Here's the drawing with two shaded views (mm, measured from the low corner). I have some questions. A direction names the side the tool comes from. Give positions to 0.01 mm unless a question says otherwise; leave off trailing zeros. Loops run counter-clockwise (first coordinate to the right, second up) from the corner with the lowest first, then second, coordinate; pieces in that order, holes last. Notation, with made-up numbers: M 15.5,8 L 55.5,8 A18 cw 55.5,21 Z; hole C 45.5,61 d6. An arc over 180 degrees is marked long. Write item = value, one per line. Start each with the question number.
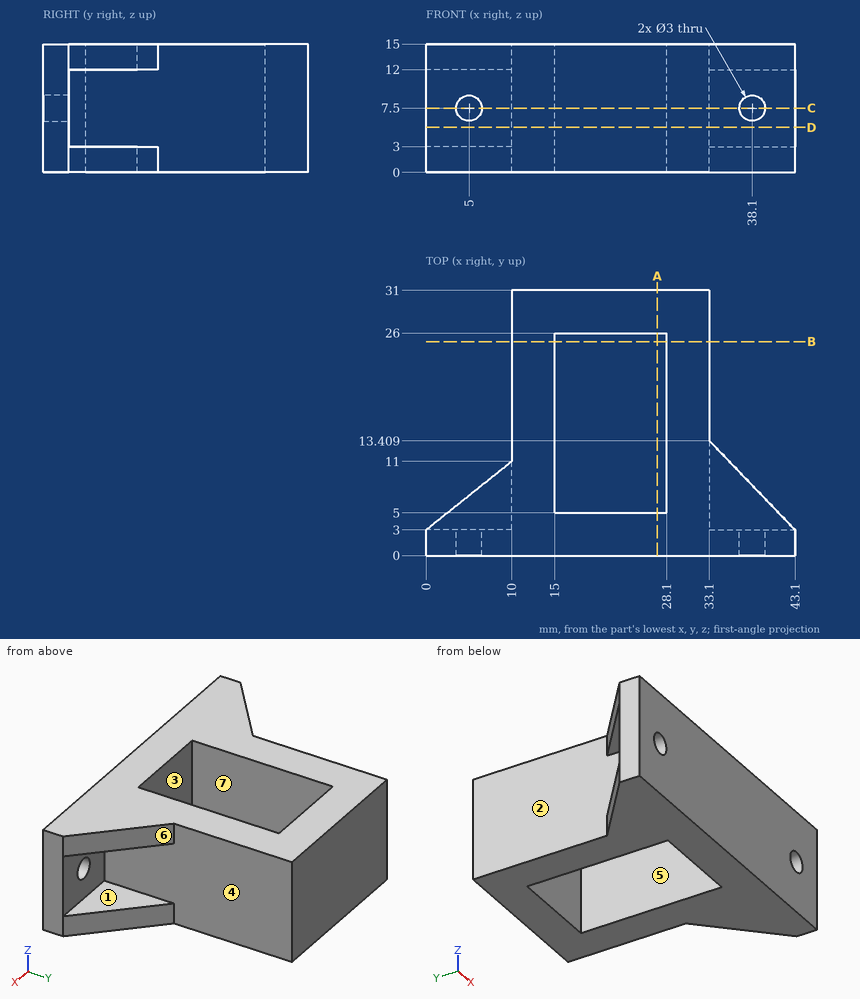
Q1. If we section it at B-B, the plane y = 25: List the corners of the cut face in (x, z) for me, then the cut area to 3 significant figures.
Q2. If I drill on line 1 along X through (y, z) = (1.5, 7.5); line 2 along Y through (x, z) = (23.5, 10.5); line 3 along X through (y, z) = (20, 8), over which ranges is the centre line in solid material (lowest first)?
Q3. On a 3-axis mill with a long thin cutter (end or side, diameter ignored), from which of +Z, -Z, +X, -X, +Y, -Y can I reach the whole of each face in a straight line? I mean the marked faces 1, 2 and 3. Say none if no direction works.
Q4. Will these pins go through, and if not, where does the flat tip stop? pin 1 (4.5 mm diameter, centred on y = 13, z = 8.5, fed in from +X); pin 2 (4.5 mm diameter, centred on x = 38, z = 9.5, fed in from +Y); pin 3 (6 mm diameter, centred on y = 15, z = 2.5, fed in from +X).
Q5. If we section it at A-A, the plane x = 27: List the corners of the cut face in (y, z) for me, then the cut area to 3 significant figures.
Q6. If we section it at D-D, the plane z = 5.25: List the corners of the cut face in (x, y) for me.
Q7. If we section it at C-C, the plane z = 7.5: List the corners of the cut face in (x, y) for me, then the cut area to 3 significant figures.
Q8. We'd pull the mould along Y, two halves only. Please class the marked faces 4, 5, 6 and 7: pulls with the +Y half, pulls with the -Y half, needs draft (parallel to the pull), parting line crosses it, or undercut.
Resolved:
q1.outline = M 10,0 L 15,0 L 15,15 L 10,15 Z; M 28.1,0 L 33.1,0 L 33.1,15 L 28.1,15 Z
q1.area = 150 mm²
q2.line_1 = 0 to 3.5, 6.5 to 36.6, 39.6 to 43.1
q2.line_2 = 0 to 5, 26 to 31
q2.line_3 = 10 to 15, 28.1 to 33.1
q3.face_1 = +X, +Y
q3.face_2 = -X, +Y
q3.face_3 = +Z, -Z
q4.pin_1 = 33.1
q4.pin_2 = 3
q4.pin_3 = 34.45
q5.outline = M 0,0 L 5,0 L 5,15 L 0,15 Z; M 26,0 L 31,0 L 31,15 L 26,15 Z
q5.area = 150 mm²
q6.outline = M 0,0 L 43.1,0 L 43.1,3 L 33.1,3 L 33.1,31 L 10,31 L 10,3 L 0,3 Z; hole M 15,5 L 28.1,5 L 28.1,26 L 15,26 Z
q7.outline = M 0,0 L 3.5,0 L 3.5,3 L 0,3 Z; M 6.5,0 L 36.6,0 L 36.6,3 L 33.1,3 L 33.1,31 L 10,31 L 10,3 L 6.5,3 Z; M 39.6,0 L 43.1,0 L 43.1,3 L 39.6,3 Z; hole M 15,5 L 28.1,5 L 28.1,26 L 15,26 Z
q7.area = 483 mm²
q8.face_4 = needs draft
q8.face_5 = undercut
q8.face_6 = pulls with the +Y half
q8.face_7 = undercut
